Work out the finished part from the listing and answer in its coordinate system (mm). Face numbers are marked on the shaded views. A direction names the side the tool comes from. Round coordinates to 2 decimals unless told otherwise and drop trailing zeros. Loops run counter-clockwise (first coordinate to the right, second up) from the corner with the lowest first, then second, coordinate; pieces in that order, holes last. Notation, with made-up numbers: M -34,89 L 10,89 A8 ccw 10,99 Z; hole C 29,84.25 d7. An arc over 180 degrees is marked long. One line per item, written item: value.
```python
from build123d import *

# Parameters (mm, degrees)
SKETCH_3_R                      = 1.7
CUT_EXTRUDE_1_DEPTH             = 10
CUT_EXTRUDE_1_DIRECTION_2_REACH = 60.902
CUT_EXTRUDE_START               = 3
SKETCH_4_R                      = 3
CUT_EXTRUDE_2_DEPTH             = 3
SKETCH_7_R                      = 3
CUT_EXTRUDE_3_DEPTH             = 10
EXTRUDE_1_DEPTH                 = 1
CHAMFER_1_SIZE                  = 1


with BuildPart() as part:
    # 草图2 → 旋转1 (revolve)
    with BuildSketch(Plane(origin=(0, 0, 0), x_dir=(0, 0, -1), z_dir=(1, 0, 0)), mode=Mode.PRIVATE) as revolve_1_sk:
        Polygon((-30, 0), (-30, 2), (-36, 2), (-36, -1.5), (-41.5, -1.5), (-41.5, -6.5), (-35, -6.5), (-35, -5.5), (-33.5, -5.5), (-33.5, 0), align=None)
    revolve(revolve_1_sk.sketch.rotate(Axis((0, 0, 0), (0, 1, 0)), 180), axis=Axis((0, 0, 0), (0, 1, 0)))

    # 草图3 → 切除-拉伸1 (cut)
    with BuildSketch(Plane(origin=(0, -1.5, 0), x_dir=(1, 0, 0), z_dir=(0, 1, 0))):
        with Locations(Location((0, 37, 0), (0, 0, 217.103674805))):
            Circle(SKETCH_3_R)
        with Locations(Location((32.04293994, 18.5, 0), (0, 0, 157.103674805))):
            Circle(SKETCH_3_R)
        with Locations(Location((32.04293994, -18.5, 0), (0, 0, 97.103674805))):
            Circle(SKETCH_3_R)
        with Locations(Location((0, -37, 0), (0, 0, 37.103674804))):
            Circle(SKETCH_3_R)
        with Locations(Location((-32.04293994, -18.5, 0), (0, 0, 82.896325196))):
            Circle(SKETCH_3_R)
        with Locations(Location((-32.04293994, 18.5, 0), (0, 0, 22.896325196))):
            Circle(SKETCH_3_R)
    extrude(amount=-CUT_EXTRUDE_1_DEPTH, mode=Mode.SUBTRACT)

    # 草图3 → 切除-拉伸1 direction 2 (cut, up to next)
    with BuildSketch(Plane(origin=(0, -1.5, 0), x_dir=(1, 0, 0), z_dir=(0, 1, 0)), mode=Mode.PRIVATE) as cut_extrude_1_direction_2_sk1:
        with Locations(Location((0, 37, 0), (0, 0, 217.103674805))):
            Circle(SKETCH_3_R)
    cut_extrude_1_direction_2_tool1 = extrude(cut_extrude_1_direction_2_sk1.sketch, amount=CUT_EXTRUDE_1_DIRECTION_2_REACH, mode=Mode.PRIVATE) & part.part
    # 草图3 → 切除-拉伸1 direction 2 (cut, up to next)
    with BuildSketch(Plane(origin=(0, -1.5, 0), x_dir=(1, 0, 0), z_dir=(0, 1, 0)), mode=Mode.PRIVATE) as cut_extrude_1_direction_2_sk2:
        with Locations(Location((32.04293994, 18.5, 0), (0, 0, 157.103674805))):
            Circle(SKETCH_3_R)
    cut_extrude_1_direction_2_tool2 = extrude(cut_extrude_1_direction_2_sk2.sketch, amount=CUT_EXTRUDE_1_DIRECTION_2_REACH, mode=Mode.PRIVATE) & part.part
    # 草图3 → 切除-拉伸1 direction 2 (cut, up to next)
    with BuildSketch(Plane(origin=(0, -1.5, 0), x_dir=(1, 0, 0), z_dir=(0, 1, 0)), mode=Mode.PRIVATE) as cut_extrude_1_direction_2_sk3:
        with Locations(Location((32.04293994, -18.5, 0), (0, 0, 97.103674805))):
            Circle(SKETCH_3_R)
    cut_extrude_1_direction_2_tool3 = extrude(cut_extrude_1_direction_2_sk3.sketch, amount=CUT_EXTRUDE_1_DIRECTION_2_REACH, mode=Mode.PRIVATE) & part.part
    # 草图3 → 切除-拉伸1 direction 2 (cut, up to next)
    with BuildSketch(Plane(origin=(0, -1.5, 0), x_dir=(1, 0, 0), z_dir=(0, 1, 0)), mode=Mode.PRIVATE) as cut_extrude_1_direction_2_sk4:
        with Locations(Location((0, -37, 0), (0, 0, 37.103674804))):
            Circle(SKETCH_3_R)
    cut_extrude_1_direction_2_tool4 = extrude(cut_extrude_1_direction_2_sk4.sketch, amount=CUT_EXTRUDE_1_DIRECTION_2_REACH, mode=Mode.PRIVATE) & part.part
    # 草图3 → 切除-拉伸1 direction 2 (cut, up to next)
    with BuildSketch(Plane(origin=(0, -1.5, 0), x_dir=(1, 0, 0), z_dir=(0, 1, 0)), mode=Mode.PRIVATE) as cut_extrude_1_direction_2_sk5:
        with Locations(Location((-32.04293994, -18.5, 0), (0, 0, 82.896325196))):
            Circle(SKETCH_3_R)
    cut_extrude_1_direction_2_tool5 = extrude(cut_extrude_1_direction_2_sk5.sketch, amount=CUT_EXTRUDE_1_DIRECTION_2_REACH, mode=Mode.PRIVATE) & part.part
    # 草图3 → 切除-拉伸1 direction 2 (cut, up to next)
    with BuildSketch(Plane(origin=(0, -1.5, 0), x_dir=(1, 0, 0), z_dir=(0, 1, 0)), mode=Mode.PRIVATE) as cut_extrude_1_direction_2_sk6:
        with Locations(Location((-32.04293994, 18.5, 0), (0, 0, 22.896325196))):
            Circle(SKETCH_3_R)
    cut_extrude_1_direction_2_tool6 = extrude(cut_extrude_1_direction_2_sk6.sketch, amount=CUT_EXTRUDE_1_DIRECTION_2_REACH, mode=Mode.PRIVATE) & part.part
    add(cut_extrude_1_direction_2_tool1.solids().sort_by_distance((0, -1.5, -37))[0], mode=Mode.SUBTRACT)
    add(cut_extrude_1_direction_2_tool2.solids().sort_by_distance((32.04294, -1.5, -18.5))[0], mode=Mode.SUBTRACT)
    add(cut_extrude_1_direction_2_tool3.solids().sort_by_distance((32.04294, -1.5, 18.5))[0], mode=Mode.SUBTRACT)
    add(cut_extrude_1_direction_2_tool4.solids().sort_by_distance((0, -1.5, 37))[0], mode=Mode.SUBTRACT)
    add(cut_extrude_1_direction_2_tool5.solids().sort_by_distance((-32.04294, -1.5, 18.5))[0], mode=Mode.SUBTRACT)
    add(cut_extrude_1_direction_2_tool6.solids().sort_by_distance((-32.04294, -1.5, -18.5))[0], mode=Mode.SUBTRACT)

    # 草图4 → 切除-拉伸2 (cut)
    with BuildSketch(Plane(origin=(0, -1.5, 0), x_dir=(1, 0, 0), z_dir=(0, 1, 0)).offset(CUT_EXTRUDE_START)):
        with Locations((0, 37)):
            Circle(SKETCH_4_R)
        with Locations((32.04293994, 18.5)):
            Circle(SKETCH_4_R)
        with Locations((32.04293994, -18.5)):
            Circle(SKETCH_4_R)
        with Locations((0, -37)):
            Circle(SKETCH_4_R)
        with Locations((-32.04293994, -18.5)):
            Circle(SKETCH_4_R)
        with Locations((-32.04293994, 18.5)):
            Circle(SKETCH_4_R)
    extrude(amount=CUT_EXTRUDE_2_DEPTH, mode=Mode.SUBTRACT)

    # 草图7 → 切除-拉伸3 (cut)
    with BuildSketch(Plane(origin=(0, -1.5, 0), x_dir=(1, 0, 0), z_dir=(0, 1, 0))):
        with Locations((32.04293994, 18.5)):
            Circle(SKETCH_7_R)
    extrude(amount=CUT_EXTRUDE_3_DEPTH, mode=Mode.SUBTRACT)

    # 草图8 → 凸台-拉伸1 (add)
    with BuildSketch(Plane(origin=(0, -1.5, 0), x_dir=(1, 0, 0), z_dir=(0, 1, 0))):
        with BuildLine():
            ThreePointArc((30.476882326, 19.161410274), (30.089095942, 19.764774357), (29.689366173, 20.360293128))
            ThreePointArc((29.689366173, 20.360293128), (29.444863729, 17), (32.477214164, 15.531598764))
            ThreePointArc((32.477214164, 15.531598764), (32.161344664, 16.175534285), (31.832709232, 16.813049186))
            ThreePointArc((31.832709232, 16.813049186), (30.570696754, 17.65), (30.476882326, 19.161410274))
        make_face()
    extrude(amount=EXTRUDE_1_DEPTH)

    # 倒角1
    # the kernel refuses this chamfer: 1 mm, written as the material it takes off along each edge
    with BuildSketch(Plane(origin=(0, 2, 0), x_dir=(0.00607290176343859, 0, 0.9999815597620647), z_dir=(-0.9999815597620647, 0, 0.00607290176343859))) as chamfer_1_piece_1:
        Polygon((36 - CHAMFER_1_SIZE, 0), (36, -CHAMFER_1_SIZE), (36, 0), align=None)
    revolve(axis=Axis((0, 2, 0), (0, 1, 0)), revolution_arc=59.304092442, mode=Mode.SUBTRACT)
    with BuildSketch(Plane(origin=(0, 2, 0), x_dir=(-0.8629729831882226, 0, 0.5052500670828455), z_dir=(-0.5052500670828455, 0, -0.8629729831882226))) as chamfer_1_piece_2:
        Polygon((36 - CHAMFER_1_SIZE, 0), (36, -CHAMFER_1_SIZE), (36, 0), align=None)
    revolve(axis=Axis((0, 2, 0), (0, 1, 0)), revolution_arc=59.304092442, mode=Mode.SUBTRACT)
    with BuildSketch(Plane(origin=(0, 2, 0), x_dir=(-0.8690458849516061, 0, -0.49473149267929145), z_dir=(0.49473149267929145, 0, -0.8690458849516061))) as chamfer_1_piece_3:
        Polygon((36 - CHAMFER_1_SIZE, 0), (36, -CHAMFER_1_SIZE), (36, 0), align=None)
    revolve(axis=Axis((0, 2, 0), (0, 1, 0)), revolution_arc=59.304092442, mode=Mode.SUBTRACT)
    with BuildSketch(Plane(origin=(0, 2, 0), x_dir=(-0.00607290176325947, 0, -0.9999815597620656), z_dir=(0.9999815597620656, 0, -0.00607290176325947))) as chamfer_1_piece_4:
        Polygon((36 - CHAMFER_1_SIZE, 0), (36, -CHAMFER_1_SIZE), (36, 0), align=None)
    revolve(axis=Axis((0, 2, 0), (0, 1, 0)), revolution_arc=59.304092442, mode=Mode.SUBTRACT)
    with BuildSketch(Plane(origin=(0, 2, 0), x_dir=(0.8629729831882953, 0, -0.5052500670827214), z_dir=(0.5052500670827214, 0, 0.8629729831882953))) as chamfer_1_piece_5:
        Polygon((36 - CHAMFER_1_SIZE, 0), (36, -CHAMFER_1_SIZE), (36, 0), align=None)
    revolve(axis=Axis((0, 2, 0), (0, 1, 0)), revolution_arc=59.304092442, mode=Mode.SUBTRACT)
    with BuildSketch(Plane(origin=(0, -1.5, 0), x_dir=(0, 0, -1), z_dir=(1, 0, 0))) as chamfer_1_piece_6:
        Polygon((41.5 - CHAMFER_1_SIZE, 0), (41.5, -CHAMFER_1_SIZE), (41.5, 0), align=None)
    revolve(axis=Axis((0, -1.5, 0), (0, 1, 0)), mode=Mode.SUBTRACT)
    with BuildSketch(Plane(origin=(0, 2, 0), x_dir=(0.8690458849516187, 0, 0.49473149267926925), z_dir=(-0.49473149267926925, 0, 0.8690458849516187))) as chamfer_1_piece_7:
        Polygon((36 - CHAMFER_1_SIZE, 0), (36, -CHAMFER_1_SIZE), (36, 0), align=None)
    revolve(axis=Axis((0, 2, 0), (0, 1, 0)), revolution_arc=59.304092442, mode=Mode.SUBTRACT)


solid = part.part
```
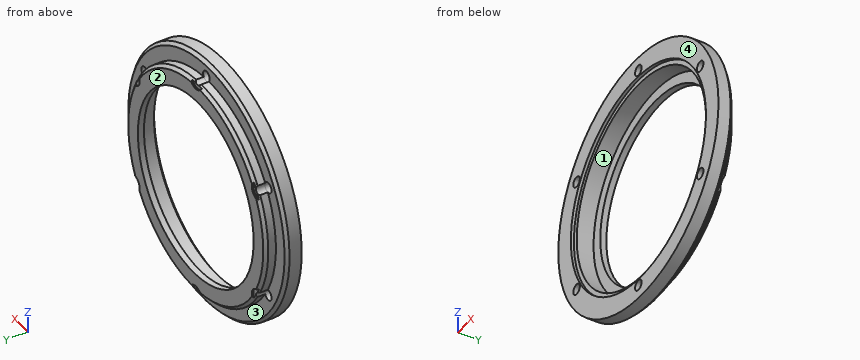
1) The mould has two halves that part along X. Classify the marked faces 1 and 2: +X half, -X half, draft (parallel to the pull), parting line (faces both ways), or undercut.
Check values:
face 1: undercut
face 2: draft
2) For the marked faces 3 and 4, determine the directions among +Z, -Z, +X, -X, +Y, -Y from which every point of the face is accessible in a straight line to the end or side of a thin tool.
Check values:
face 3: +Y
face 4: +Z, -Z, +X, -X, -Y
3) Find section A-A (z = 0). Give the vertices of the cut face in (x, y).
Check values:
outline: M -41.5,-6.5 L -35,-6.5 L -35,-5.5 L -33.5,-5.5 L -33.5,0 L -30,0 L -30,2 L -35,2 L -36,1 L -36,-1.5 L -40.5,-1.5 L -41.5,-2.5 Z; M 30,0 L 33.5,0 L 33.5,-5.5 L 35,-5.5 L 35,-6.5 L 41.5,-6.5 L 41.5,-2.5 L 40.5,-1.5 L 36,-1.5 L 36,1 L 35,2 L 30,2 Z
4) Find the intervals of material crossed by probe 1 along X at (y, z) = (-3.5, -20); probe 2 along Z at (x, y) = (17, -4.25); probe 3 along Z at (x, y) = (-8.5, 1.5), in increasing order. Write a range as from..to.
Check values:
probe 1: -36.36..-32.84, -31.24..-26.87, 26.87..31.24, 32.84..36.36
probe 2: -37.86..-28.87, 28.87..37.86
probe 3: -34.47..-28.77, 28.77..34.47
5) Each of these flat-tipped pins is pushed along its axis until it touches: pin 1 (3 mm diameter, centred on x = -30.5, z = 18, fed in from +Y); pin 2 (4 mm diameter, centred on x = 32.04, z = 18.5, fed in from +Y); pin 3 (1.5 mm diameter, centred on y = -5, z = -11, fed in from +X); pin 4 (1.5 mm diameter, centred on y = -5.5, z = 7, fed in from -X). Where does it stop, or does it pass through?
Check values:
pin 1: y = 2
pin 2: y = 1.5
pin 3: x = 40.21
pin 4: x = -41.03
